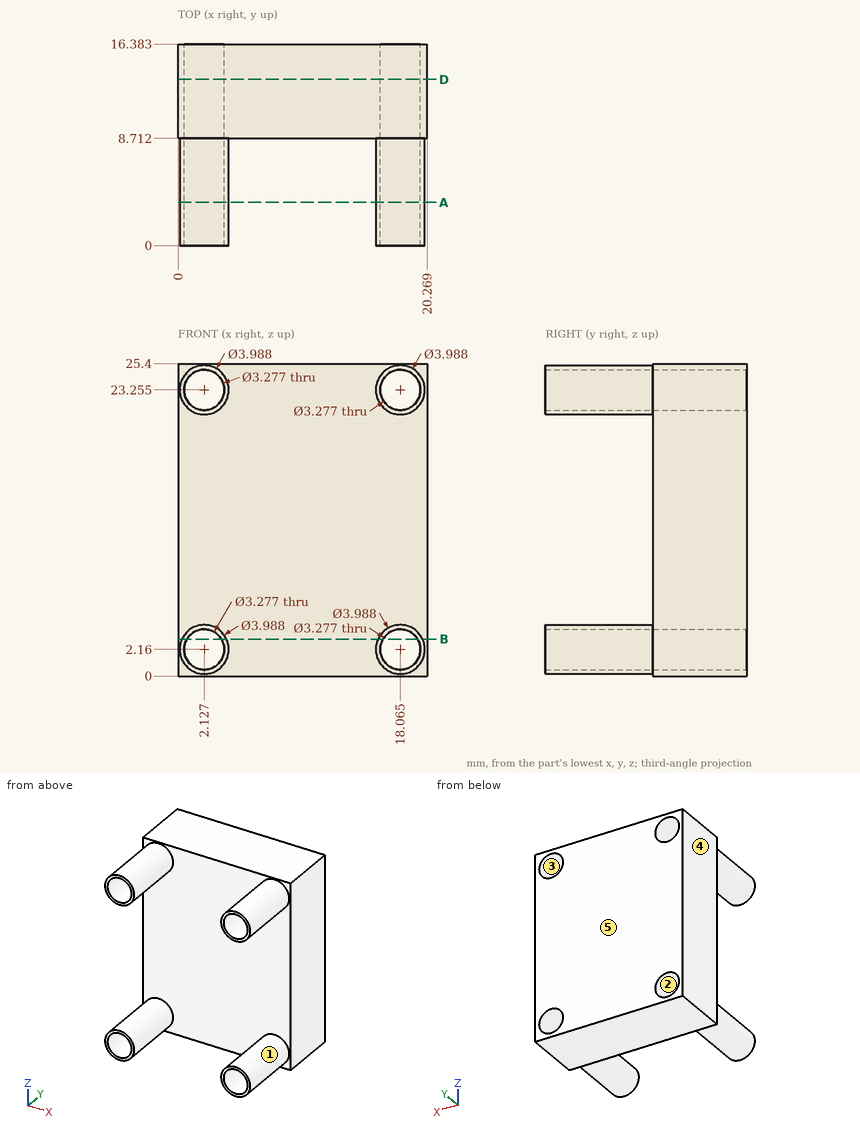
Here's the drawing with two shaded views (mm, measured from the low corner). I have some questions. A direction names the side the tool comes from. Round coordinates to 2 decimals unless told otherwise and drop trailing zeros. Write each loop counter-clockwise with the first axis right and the second up, starting at its lowest first coordinate (ties: lowest second). Pieces come first, ordered by that corner, then holes.
(1) For pin 1 (1.5 mm diameter, centred on x = 18, y = 2.5, fed in from +Z), with a flat end and sliding along its axis, tell me the tip position at first contact or that it passes through.
Findings below:
pin 1: stops at z = 25.25
(2) Suppose I cut it at A-A on y = 3.5. Write out the boundary of the cut face in (x, z) (1 decimal).
Findings below:
outline: circle Ø4 at (2.1, 2.2); circle Ø4 at (2.1, 23.3); circle Ø4 at (18.1, 2.2); circle Ø4 at (18.1, 23.3); hole circle Ø3.3 at (2.1, 2.2); hole circle Ø3.3 at (2.1, 23.3); hole circle Ø3.3 at (18.1, 2.2); hole circle Ø3.3 at (18.1, 23.3)
(3) Which directions (+Z, -Z, +X, -X, +Y, -Y) give clear straight access to the entire face, cutting with the end or side of a thin tool? Please do the marked faces 1 and 2.
Findings below:
face 1: -Y
face 2: +Y, -Y
(4) Suppose I cut it at D-D on y = 13.5. Write out the boundary of the cut face in (x, z) (1 decimal), and give its area (3 significant figures).
Findings below:
outline: (0, 0) - (20.3, 0) - (20.3, 25.4) - (0, 25.4) - close; hole circle Ø3.3 at (2.1, 2.2); hole circle Ø3.3 at (2.1, 23.3); hole circle Ø3.3 at (18.1, 2.2); hole circle Ø3.3 at (18.1, 23.3)
area: 481 mm2
(5) Thinking about a two-plate mould opening in X: for the marked faces 3, 4 and 5, which applies, +X half, -X half, draft (parallel to the pull), parting line (faces both ways), or undercut?
Findings below:
face 3: undercut
face 4: -X half
face 5: draft
(6) Suppose I cut it at B-B on z = 3. State how many separate pieces and enclosed holes the cut face has, and give its area (3 significant figures).
Findings below:
separate pieces: 3
enclosed holes: 0
area: 126 mm2
(7) If I drill on probe 1 along X at (y, z) = (14.25, 1) (1 decimal); probe 2 along Z at (x, y) = (2.75, 9.5) (1 decimal); probe 3 along X at (y, z) = (6, 23.5) (1 decimal), over which ranges is the centre line in solid material (lowest first)?
Findings below:
probe 1: x = 0 to 1, 3.3 to 16.9, 19.2 to 20.3
probe 2: z = 0 to 0.6, 3.7 to 21.7, 24.8 to 25.4
probe 3: x = 0.1 to 0.5, 3.7 to 4.1, 16.1 to 16.4, 19.7 to 20
